```python
from build123d import *

# Parameters (mm, degrees)
F13_W     = 152.3095369339
F13_H     = 45.384734869
F1_DEPTH  = 25.4
F2_DEPTH  = 25.4
F4_R      = 10.680963323
F5_DEPTH  = 25.401
F6_R      = 12.4666506347
F15_DEPTH = 25.401
F3_W      = 67.3640072346
F3_H      = 26.1916220188
F16_DEPTH = 25.4
F17_DEPTH = 67.4096792936
F8_R      = 10.4571880182
F10_DEPTH = 36.4030317793
F11_R     = 5.1214106797
F12_DEPTH = 132.9530260163


with BuildPart() as f1:
    # F13 (on Front) → F1 (new body)
    with BuildSketch(Plane.XZ):
        with Locations((0.9222924709, 0.6138533354)):
            Rectangle(F13_W, F13_H)
    extrude(amount=F1_DEPTH)

    # F14 (on face) + F0 (on face) → F2 (join)
    with BuildSketch(Plane.XZ):
        with BuildLine():
            Line((-75.232475996, -22.0671208814), (-75.232475996, 22.0671208814))
            ThreePointArc((-75.232475996, 22.0671208814), (-98.2022533394, 0), (-75.232475996, -22.0671208814))
        make_face()
    with BuildSketch(Plane.XZ):
        with BuildLine():
            ThreePointArc((72.386937855, -22.0785140991), (91.0472381253, -17.3936843382), (99.270022399, 0))
            ThreePointArc((99.270022399, 0), (92.7885691568, 15.8037323084), (77.0770609379, 22.5056499815))
            Line((77.0770609379, 22.5056499815), (77.0770609379, -22.0785140991))
            Line((77.0770609379, -22.0785140991), (72.386937855, -22.0785140991))
        make_face()
    extrude(amount=F2_DEPTH)

    # F4 (on face) → F5 (cut, through all)
    with BuildSketch(Plane.XZ.offset(25.4)):
        with Locations((-63.1323754787, 0)):
            Circle(F4_R)
    extrude(amount=-F5_DEPTH, mode=Mode.SUBTRACT)

    # F6 (on face) → F15 (cut, through all)
    with BuildSketch(Plane.XZ.offset(25.4)):
        with Locations((63.0310773849, 0)):
            Circle(F6_R)
    extrude(amount=-F15_DEPTH, mode=Mode.SUBTRACT)

    # F3 (on face) → F16 (join)
    with BuildSketch(Plane.XZ.offset(25.4)):
        Rectangle(F3_W, F3_H)
    extrude(amount=F16_DEPTH)

    # F7 (on face) → F17 (join)
    with BuildSketch(Plane(origin=(-33.6820036173, 0, 0), x_dir=(0, -1, 0), z_dir=(-1, 0, 0))):
        with BuildLine():
            ThreePointArc((50.8, -12.9561868231), (59.961407561, -9.161407561), (63.7561868231, 0))
            ThreePointArc((63.7561868231, 0), (59.961407561, 9.161407561), (50.8, 12.9561868231))
            Line((50.8, 12.9561868231), (50.8, -12.9561868231))
        make_face()
    extrude(amount=-F17_DEPTH)

    # F8 (on face) + F9 (on face) → F10 (cut, through all)
    with BuildSketch(Plane(origin=(0, 0, -13.0958110094), x_dir=(1, 0, 0), z_dir=(0, 0, -1))):
        with Locations((0, 38.6807024479)):
            Circle(F8_R)
    with BuildSketch(Plane(origin=(0, 0, -13.0958110094), x_dir=(1, 0, 0), z_dir=(0, 0, -1))):
        with BuildLine():
            ThreePointArc((-10.4190511629, 39.5729771324), (0.2211320485, 49.1355521295), (10.4474613547, 39.1316264868))
            Line((10.4474613547, 39.1316264868), (10.4537252337, 39.1316264868))
            Line((10.4537252337, 39.1316264868), (10.4537252337, 65.8641159534))
            Line((10.4537252337, 65.8641159534), (-10.4190511629, 65.8641159534))
            Line((-10.4190511629, 65.8641159534), (-10.4190511629, 39.5729771324))
        make_face()
    extrude(amount=-F10_DEPTH, mode=Mode.SUBTRACT)

    # F11 (on face) → F12 (cut, through all)
    with BuildSketch(Plane(origin=(-33.6820036173, 0, 0), x_dir=(0, -1, 0), z_dir=(-1, 0, 0))):
        with Locations((50.8, 0)):
            Circle(F11_R)
    extrude(amount=-F12_DEPTH, mode=Mode.SUBTRACT)


solid = f1.part
```
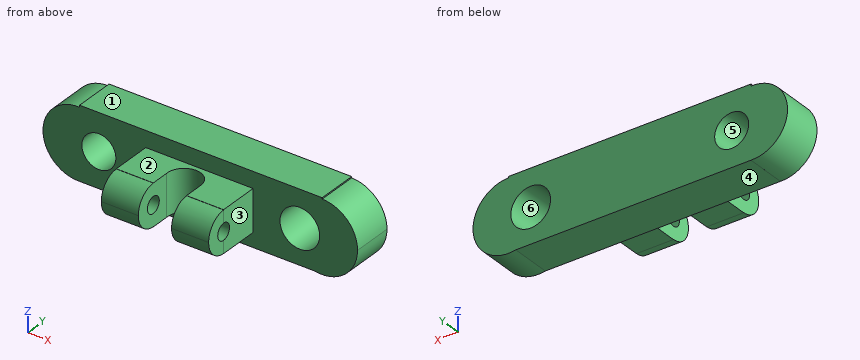
CAD build for the part. Positions are in the model's coordinates, mm. Face numbers are marked on the shaded views. A direction names the side the tool comes from. Round coordinates to 2 decimals unless told otherwise and drop trailing zeros. Loops run counter-clockwise (first coordinate to the right, second up) from the corner with the lowest first, then second, coordinate; pieces in that order, holes last. Notation, with made-up numbers: M 42,-36.5 L 57,-36.5 A33 cw 57,-2.5 Z; hole C 9,-11.5 d5. An arc over 180 degrees is marked long. Use a Markdown table: item, result. Add a question column.
(1) Cut at C-C (y = -12). State how many separate pieces and enclosed holes the cut face has, and give its area (3 significant figures).
(2) Flat gauge pins, fed straight in: pin 1 (12 mm diameter, centred on y = -15, z = 11, fed in from +X); pin 2 (6 mm diameter, centred on y = -48.5, z = -14.5, fed in from -X); pin 3 (14.5 mm diameter, centred on y = -57, z = 4.5, fed in from +X). Where does each tip first touch, or does it go through?
(3) Cut at B-B (x = 0). Give the cut face in (y, z), and give its area (3 significant figures).
(4) Cut at D-D (y = -58.5). Give the cut face in (x, z), and give its area (3 significant figures).
(5) Pull direction Z, two halves, no side cores. Call the marked faces 3, 4, 5 and 6: +Z half, -Z half, draft (parallel to the pull), parting line (faces both ways), or undercut.
(6) Which spindle directions (+Z, -Z, +X, -X, +Y, -Y) get a long thin tool onto all of the face, cutting with end or side? Do the marked faces 1 and 2. Say none if no direction does.
(7) Drill centre lines: line 1 (X direction, y = -53, z = -6.5); line 2 (Y direction, x = -41, z = -8.5); line 3 (Z direction, x = -25, y = -54.5). Where is each one in solid material? Low to high.
(8) Cut at A-A (y = -30.5). Give the cut face in (x, z).
Geometry says:
| question | item | result |
|---|---|---|
| 1 | separate pieces | 1 |
| 1 | enclosed holes | 2 |
| 1 | area | 7,650 mm² |
| 2 | pin 1 | stops at x = 98.71 |
| 2 | pin 2 | stops at x = -33.68 |
| 2 | pin 3 | stops at x = 33.73 |
| 3 | outline | M -28.22,-13.1 L -25.4,-13.1 L -25.4,-22.08 L 0,-22.08 L 0,23.31 L -25.4,23.31 L -25.4,13.1 L -28.22,13.1 Z |
| 3 | area | 1,230 mm² |
| 4 | outline | M -33.68,-10.42 L -10.42,-10.42 L -10.42,10.42 L -33.68,10.42 Z; M 10.45,-10.42 L 33.73,-10.42 L 33.73,10.42 L 10.45,10.42 Z |
| 4 | area | 970 mm² |
| 5 | face 3 | draft |
| 5 | face 4 | -Z half |
| 5 | face 5 | undercut |
| 5 | face 6 | undercut |
| 6 | face 1 | +Z, +X, -X, +Y, -Y |
| 6 | face 2 | +Z, +X, -X, -Y |
| 7 | line 1 | x = -33.68 to -10.42, 10.45 to 33.73 |
| 7 | line 2 | y = -25.4 to 0 |
| 7 | line 3 | z = -12.42 to -3.54, 3.54 to 12.42 |
| 8 | outline | M -33.68,-13.1 L -6.51,-13.1 L -6.51,13.1 L -33.68,13.1 Z; M 6.51,-13.1 L 33.68,-13.1 L 33.68,13.1 L 6.51,13.1 Z |
